from build123d import *

# Parameters (mm, degrees)
BOSS_EXTRUDE2_DEPTH = 200.914
CUT_EXTRUDE1_DEPTH  = 26.4
CUT_EXTRUDE2_DEPTH  = 26.4


with BuildPart() as part:
    # Sketch2 → Boss-Extrude2 (new body)
    with BuildSketch(Plane(origin=(0, 0, 0), x_dir=(1, 0, 0), z_dir=(0, 1, 0))):
        Polygon((0, 0), (0, 25.4), (1.5875, 25.4), (1.5875, 1.5875), (25.4, 1.5875), (25.4, 0), align=None)
    extrude(amount=BOSS_EXTRUDE2_DEPTH)

    # Sketch4 → Cut-Extrude1 (cut, through all)
    with BuildSketch(Plane.XY):
        Polygon((0, 200.914), (25.4, 175.514), (25.4, 200.914), align=None)
    extrude(amount=-CUT_EXTRUDE1_DEPTH, mode=Mode.SUBTRACT)

    # Sketch5 → Cut-Extrude2 (cut, through all)
    with BuildSketch(Plane.XY):
        Polygon((0, 0), (25.4, 25.4), (25.4, 0), align=None)
    extrude(amount=-CUT_EXTRUDE2_DEPTH, mode=Mode.SUBTRACT)


solid = part.part
Work out the finished part from the listing and answer in its coordinate system (mm). A direction names the side the tool comes from. Round coordinates to 2 decimals unless told otherwise and drop trailing zeros. Loops run counter-clockwise (first coordinate to the right, second up) from the corner with the lowest first, then second, coordinate; pieces in that order, holes last. Notation, with made-up numbers: (-23.75, 33.5) -> (21.25, 33.5) arc R6 ccw to (21.25, 40.5) -> close; hole circle Ø3 at (74, 32.25). An arc over 180 degrees is marked (long way). Use one line per item in the form item = value.
(1) Find section A-A on y = 144.5. Give the vertices of the cut face in (x, z), then the cut area to 3 significant figures.
Answer list:
outline = (0, -25.4) -> (1.59, -25.4) -> (1.59, -1.59) -> (25.4, -1.59) -> (25.4, 0) -> (0, 0) -> close
area = 78.1 mm2
(2) Flat-ended cylindrical pins translate along their axes: P1, Ø4, axis at y = 133.5, z = -21, coming from the +X side; P2, Ø8, axis at x = 19.5, y = 173, coming from the -Z side. Find the tip coordinate at first contact, or state that the pin passes through.
Answer list:
P1 = 1.59
P2 = -1.59
(3) Find section B-B on z = -12. Give the vertices of the cut face in (x, y).
Answer list:
outline = (0, 0) -> (1.59, 1.59) -> (1.59, 199.33) -> (0, 200.91) -> close
(4) Straight lines are drawn through the part: line 1 (Z direction, x = 3.5, y = 189.5); line 2 (X direction, y = 113, z = -23.25). For each, find the intervals that lie inside material, in ascending order.
Answer list:
line_1 = -1.59 to 0
line_2 = 0 to 1.59
(5) A tool of negligible diameter and unlimited length cuts with its end or side. For faces 1 (the flat face through (13, 99, -1.588)), 2 (the flat face through (0, 99, -13)), from which of +Z, -Z, +X, -X, +Y, -Y can it reach the whole face along a straight path? Write none if from no direction.
Answer list:
face_1 = -Z, +X, +Y, -Y
face_2 = +Z, -Z, -X, +Y, -Y
(6) Find section C-C on x = 7.25. Give the vertices of the cut face in (y, z).
Answer list:
outline = (7.25, -1.59) -> (193.66, -1.59) -> (193.66, 0) -> (7.25, 0) -> close
